Input: part model. Units: mm. Frame: model coordinates. A direction names the side the tool comes from. Round coordinates to 2 decimals unless told otherwise and drop trailing zeros. Loops run counter-clockwise (first coordinate to the right, second up) from the corner with the lowest first, then second, coordinate; pieces in that order, holes last. Notation, with made-up numbers: (5.25, 66) -> (64.25, 66) arc R14 ccw to (64.25, 70) -> close; hole circle Ø8 at (85, 68.25). An arc over 180 degrees is marked (long way). One line per question, with ' | ' between items. Start each with the question number.
Q1. Mould query, pull axis Z, two halves, no side actions, for faces 1 (the face through (-11.43, -3, 13)), 2 (the face through (-18, 0, 14)), 3 (the face through (-17.43, 59.88, 27.95)). Classes: pulls with the +Z half, pulls with the -Z half, needs draft (parallel to the pull), parting line crosses it, or undercut.
Q2. Cut plane B-B on z = 11. Return loops of the section in (x, y) (3 decimals).
Q3. Material intervals for L1, parallel to Z at x = -19.5, y = 7 (3 decimals); L2, parallel to Z at x = -14, y = 40 (3 decimals); L3, parallel to Y at x = -17, z = 8.5, sorted ascending.
Q4. Access query for faces 4 (the face through (-18, 70.559, 30)), 5 (the face through (-8.946, -3.131, 21.058)), 6 (the face through (-17, 46, 33.782)), 7 (the face through (-17, 65, 25.972)). Directions: +Z, -Z, +X, -X, +Y, -Y. A direction counts if a zero-diameter tool reaches every point of the face in a straight line with its end or side. Return the directions, or none.
Q5. Contact query for flat-ended pins moving along their axis: P1, Ø1, axis at x = -18.5, z = 30.5, coming from the +Y side (3 decimals); P2, Ø2, axis at x = -9.5, y = 33, coming from the -Z side (3 decimals); P3, Ø0.6, axis at x = -15.5, z = 32.5, coming from the +Y side; P4, Ø0.6, axis at x = -26, z = 34.5, coming from the +Y side (3 decimals). Output: stop coordinate, or through.
Q6. Cut plane A-A on y = 42.5. Return loops of the section in (x, z) (3 decimals).
from build123d import *

# Parameters (mm, degrees)
F0_W      = 17.4625
F0_H      = 34.925
F1_DEPTH  = 6.35
F2_W      = 34.925
F2_H      = 6.35
F3_DEPTH  = 73.025
F5_DEPTH  = 3.175
F7_DEPTH  = 3.175
F8_W      = 34.925
F8_H      = 3.175
F9_DEPTH  = 17.78
F10_W     = 34.925
F10_H     = 1.143
F10_H_2   = 0.889
F11_DEPTH = 18.1102
F12_W     = 10.16
F12_H     = 15.24
F13_DEPTH = 25.4
F14_W     = 5.0834602067
F14_H     = 0.7943399184
F14_H_2   = 4.191
F15_DEPTH = 12.7
F17_DEPTH = 5.7404
F18_R     = 1.58749
F19_W     = 5.0834602067
F19_H     = 0.7931600816
F20_DEPTH = 12.7


# Not quite as in the source:
# - a fillet or chamfer is up to 0.001 mm smaller than in the source, because OpenCascade refuses the exact size
# - a feature names something its author has since deleted; it is built from what else it names


with BuildPart() as f1:
    # F0 (on Front) → F1 (new body)
    with BuildSketch(Plane.XZ):
        with Locations((-8.73125, 17.4625)):
            Rectangle(F0_W, F0_H)
        with BuildLine():
            ThreePointArc((-11.43, 18.5185023174), (-8.89, 21.0585023174), (-6.35, 18.5185023174))
            Line((-6.35, 18.5185023174), (-6.35, 8.2149775699))
            ThreePointArc((-6.35, 8.2149775699), (-8.89, 5.6749775699), (-11.43, 8.2149775699))
            Line((-11.43, 8.2149775699), (-11.43, 18.5185023174))
        make_face(mode=Mode.SUBTRACT)
        with Locations((-26.19375, 17.4625)):
            Rectangle(F0_W, F0_H)
        with BuildLine():
            Line((-23.495, 18.5185023174), (-23.495, 8.2149775699))
            ThreePointArc((-23.495, 8.2149775699), (-26.0048819907, 5.6751561381), (-28.5742857524, 8.154745786))
            ThreePointArc((-28.5742857524, 8.154745786), (-28.5748214318, 8.1848595606), (-28.575, 8.2149775699))
            Line((-28.575, 8.2149775699), (-28.575, 18.5185023174))
            ThreePointArc((-28.575, 18.5185023174), (-26.035, 21.0585023174), (-23.495, 18.5185023174))
        make_face(mode=Mode.SUBTRACT)
    extrude(amount=F1_DEPTH)

    # F2 (on face) → F3 (join)
    with BuildSketch(Plane(origin=(0, 0, 0), x_dir=(-1, 0, 0), z_dir=(0, 1, 0))):
        with Locations((17.4625, 31.75)):
            Rectangle(F2_W, F2_H)
    extrude(amount=F3_DEPTH)

    # F4 (on face) → F5 (join)
    with BuildSketch(Plane.YZ):
        Polygon((0, 28.575), (0, 14.2875), (36.5125, 28.575), align=None)
    extrude(amount=-F5_DEPTH)

    # F6 (on face) → F7 (join)
    with BuildSketch(Plane(origin=(-34.925, 0, 0), x_dir=(0, -1, 0), z_dir=(-1, 0, 0))):
        Polygon((-36.5125, 28.575), (0, 14.2875), (0, 28.575), align=None)
    extrude(amount=-F7_DEPTH)

    # F8 (on face) → F9 (cut)
    with BuildSketch(Plane(origin=(0, 73.025, 0), x_dir=(-1, 0, 0), z_dir=(0, 1, 0))):
        with Locations((17.4625, 33.3375)):
            Rectangle(F8_W, F8_H)
    extrude(amount=-F9_DEPTH, mode=Mode.SUBTRACT)

    # F10 (on face) → F11 (cut)
    with BuildSketch(Plane(origin=(0, 55.245, 0), x_dir=(-1, 0, 0), z_dir=(0, 1, 0))):
        with Locations((17.4625, 33.2105)):
            Rectangle(F10_W, F10_H)
        with Locations((17.4625, 32.1945)):
            Rectangle(F10_W, F10_H_2)
    extrude(amount=-F11_DEPTH, mode=Mode.SUBTRACT)

    # F12 (on face) → F13 (cut)
    with BuildSketch(Plane.XY.offset(31.75)):
        with Locations((-17.4625, 62.9390887916)):
            Rectangle(F12_W, F12_H)
    extrude(amount=-F13_DEPTH, mode=Mode.SUBTRACT)

    # F14 (on face) → F15 (join)
    with BuildSketch(Plane(origin=(0, 55.3190887916, 0), x_dir=(-1, 0, 0), z_dir=(0, 1, 0))):
        with Locations((17.4607698967, 30.5596699592)):
            Rectangle(F14_W, F14_H)
        with Locations((17.4607698967, 28.067)):
            Rectangle(F14_W, F14_H_2)
    extrude(amount=F15_DEPTH)

    # F16 (on face) → F17 (cut)
    with BuildSketch(Plane.YZ.offset(-14.9190397933)):
        Polygon((68.0190887916, 28.4641699592), (65.845951438, 25.9715), (67.369951438, 25.9715), (68.0190887916, 25.9715), align=None)
        Polygon((55.3190887916, 25.9715), (62.7900138497, 25.9715), (64.3140138497, 25.9715), (55.3190887916, 29.9881699592), (55.3190887916, 28.575), align=None)
    extrude(amount=-F17_DEPTH, mode=Mode.SUBTRACT)

    # F18 (radius 1.5875 in the source; OpenCascade refuses exactly that, so slightly less here)
    f18_edges = [f1.edges().sort_by_distance(p)[0] for p in [
        (-17.4625, 73.025, 31.75),
        (-17.4625, 73.025, 28.575),
    ]]
    fillet(f18_edges, radius=F18_R)

    # F19 (on face) → F20 (join)
    with BuildSketch(Plane(origin=(0, 55.3190887916, 0), x_dir=(-1, 0, 0), z_dir=(0, 1, 0))):
        with Locations((17.4607698967, 31.3534199592)):
            Rectangle(F19_W, F19_H)
    extrude(amount=F20_DEPTH)


solid = f1.part
Results:
1) face 1: undercut | face 2: needs draft | face 3: pulls with the -Z half
2) outline: (-34.925, -6.35) -> (-28.575, -6.35) -> (-28.575, 0) -> (-34.925, 0) -> close; (-23.495, -6.35) -> (-11.43, -6.35) -> (-11.43, 0) -> (-23.495, 0) -> close; (-6.35, -6.35) -> (0, -6.35) -> (0, 0) -> (-6.35, 0) -> close
3) L1: 28.575 to 34.925 | L2: 28.575 to 31.75, 33.782 to 34.925 | L3: -6.35 to 0
4) face 4: +Z, -Z | face 5: +Y, -Y | face 6: +X, -X, +Y | face 7: -Z, +X, -X, +Y
5) P1: y = 73.025 | P2: z = 28.575 | P3: y = 37.13 | P4: y = 55.245
6) outline: (-34.925, 28.575) -> (0, 28.575) -> (0, 31.75) -> (-34.925, 31.75) -> close; (-34.925, 33.782) -> (0, 33.782) -> (0, 34.925) -> (-34.925, 34.925) -> close
